Job drawing, mm, ordinate dimensions from the low corner. One solid piece. A direction names the side the tool comes from. Give positions to 0.01 mm unless a question says otherwise; leave off trailing zeros. Write each loop counter-clockwise with the first axis right and the second up, starting at its lowest first coordinate (ties: lowest second). Pieces come first, ordered by that corner, then holes. Notation, with made-up numbers: (-23, 84) - (-7, 84) arc R24 cw to (-7, 114) - close; hole circle Ø3 at (-16.5, 77.5). An arc over 180 degrees is marked (long way). Put each result on its own line as item: value. Start each with the question number.
1. Tool access for the marked faces 1 and 2: list every direction of +Z, -Z, +X, -X, +Y, -Y with a clear straight run to the whole face (end or side of a thin tool).
2. Drop flat-ended pins along their axis: pin 1 (6 mm diameter, centred on x = 9, z = 4.5, fed in from +Y); pin 2 (1.2 mm diameter, centred on x = 6.5, y = 2.5, fed in from -Z); pin 3 (2 mm diameter, centred on x = 11.5, z = 14, fed in from +Y); pin 4 (0.9 mm diameter, centred on y = 3, z = 2, fed in from -X). Give the stop position or say it passes through.
3. Cut at B-B on y = 2.25. List the corners of the cut face in (x, z).
4. Cut at D-D on z = 20. List the corners of the cut face in (x, y), and give its area (3 significant figures).
5. Cut at C-C on x = 6.5. List the corners of the cut face in (y, z), and give its area (3 significant figures).
6. Wall check: line 1 (Y direction, x = 6.25, z = 24.5); line 2 (Z direction, x = 11.5, y = 12.25); line 3 (X direction, y = 10, z = 17.5). Give the ranges that are in metal, low to high.
7. Cut at A-A on y = 10.2. List the corners of the cut face in (x, z).
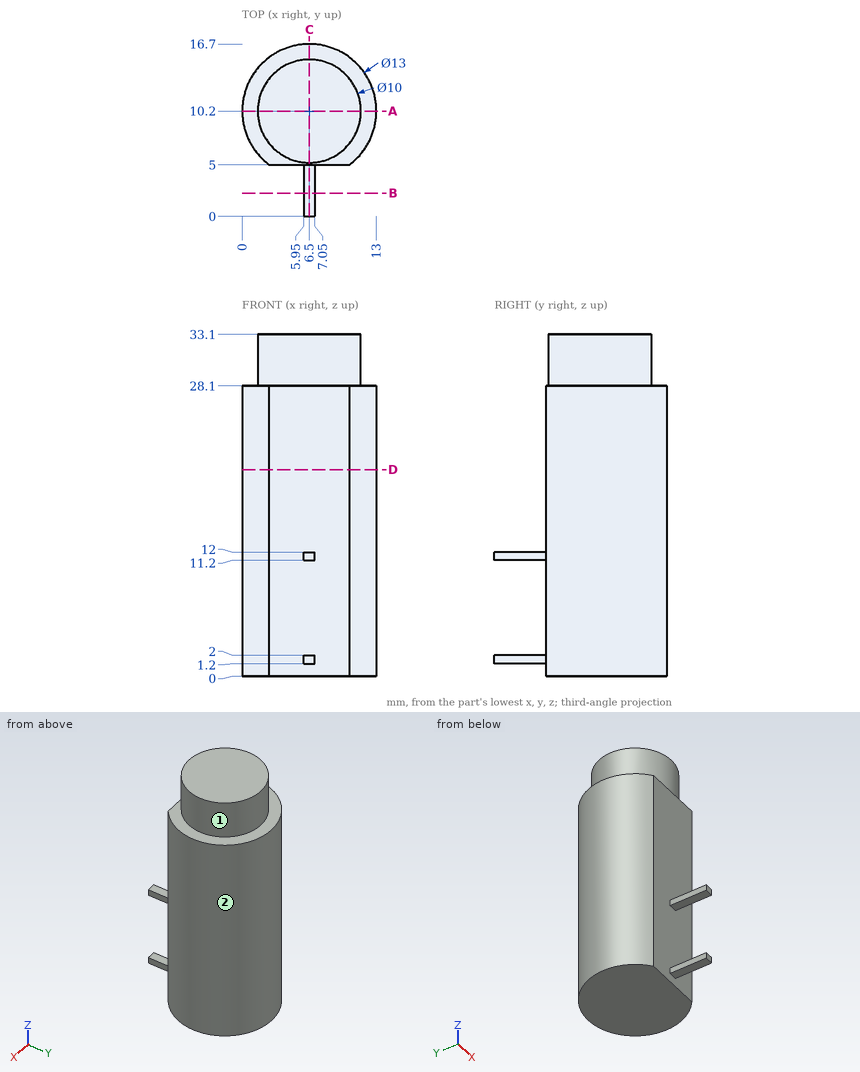
Report:
1. face 1: +Z
1. face 2: +Z, -Z
2. pin 1: stops at y = 16.7
2. pin 2: stops at z = 1.2
2. pin 3: stops at y = 15.32
2. pin 4: stops at x = 5.95
3. outline: (5.95, 1.2) - (7.05, 1.2) - (7.05, 2) - (5.95, 2) - close; (5.95, 11.2) - (7.05, 11.2) - (7.05, 12) - (5.95, 12) - close
4. outline: (2.6, 5) - (10.4, 5) arc R6.5 ccw (long way) to start
4. area: 126 mm²
5. outline: (0, 1.2) - (5, 1.2) - (5, 0) - (16.7, 0) - (16.7, 28.1) - (15.2, 28.1) - (15.2, 33.1) - (5.2, 33.1) - (5.2, 28.1) - (5, 28.1) - (5, 12) - (0, 12) - (0, 11.2) - (5, 11.2) - (5, 2) - (0, 2) - close
5. area: 387 mm²
6. line 1: y = 5 to 16.7
6. line 2: z = 0 to 28.1
6. line 3: x = 0 to 13
7. outline: (0, 0) - (13, 0) - (13, 28.1) - (11.5, 28.1) - (11.5, 33.1) - (1.5, 33.1) - (1.5, 28.1) - (0, 28.1) - close
